Build history of the part. All positions in model axes, mm. Face numbers are marked on the shaded views. A direction names the side the tool comes from. Round coordinates to 2 decimals unless told otherwise and drop trailing zeros. Write each loop counter-clockwise with the first axis right and the second up, starting at its lowest first coordinate (ties: lowest second). Pieces come first, ordered by that corner, then holes. Notation, with made-up numbers: (20.25, 64.5) - (48.25, 64.5) arc R28 cw to (48.25, 90.5) - close; hole circle Ø2 at (24, 41.25). An arc over 180 degrees is marked (long way). One line per question, with ' | ' between items.
from build123d import *

# Parameters (mm, degrees)
F0_R     = 42
F0_R_2   = 26
F1_DEPTH = 2.5
F2_R     = 2
F3_R     = 26.5
F4_DEPTH = 45
F5_R     = 2.5
F6_T     = -0.5


# Not quite as in the source:
# - a shell that OpenCascade refuses in one call is made with other operations: the cavity is built on its own and cut out


with BuildPart() as f1:
    # F0 (on Top) → F1 (new body)
    with BuildSketch(Plane.XY):
        Circle(F0_R)
        Circle(F0_R_2, mode=Mode.SUBTRACT)
    extrude(amount=F1_DEPTH)

    # F2
    f2_edges = [f1.edges().sort_by_distance(p)[0] for p in [
        (-42, 0, 2.5),
    ]]
    fillet(f2_edges, radius=F2_R)

    # F3 (on face) → F4 (join)
    with BuildSketch(Plane(origin=(0, 0, 0), x_dir=(1, 0, 0), z_dir=(0, 0, -1))):
        Circle(F3_R)
    extrude(amount=F4_DEPTH)

    # F5
    f5_edges = [f1.edges().sort_by_distance(p)[0] for p in [
        (-26.5, 0, -45),
    ]]
    fillet(f5_edges, radius=F5_R)

    # F6: a shell. OpenCascade refuses it in one call, so the cavity is built on its own and cut out:
    # the body offset inwards by the wall thickness, plus a prism from it out through each open face.
    f6_core = offset(f1.part, amount=F6_T, kind=Kind.INTERSECTION, mode=Mode.PRIVATE)
    f6_exits = [f6_core.faces().sort_by_distance(p)[0] for p in [
        (0, 0, -0.5),
    ]]
    add(f6_core, mode=Mode.SUBTRACT)
    extrude(f6_exits, amount=-F6_T, mode=Mode.SUBTRACT)


solid = f1.part
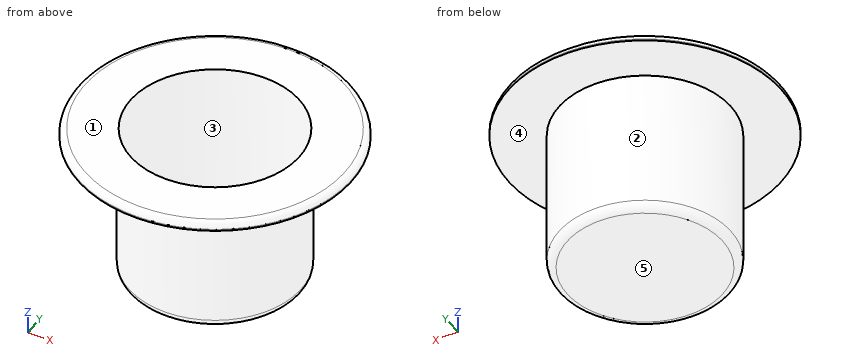
Q1. Pull direction X, two halves, no side cores. Call the marked faces 1, 2 and 3: +X half, -X half, draft (parallel to the pull), parting line (faces both ways), or undercut.
Found:
face 1: draft | face 2: parting line | face 3: undercut
Q2. Drill centre lines: L1, parallel to Y at x = 0, z = -18.5; L2, parallel to Z at x = 19, y = -19.5. Where is each one in solid material? Low to high. Write a range as from..to.
Found:
L1: -26.5..-26, 26..26.5 | L2: 0..2.5
Q3. Drop flat-ended pins along their axis: pin 1 (8 mm diameter, centred on y = 23.5, z = -9.5, fed in from -X); pin 2 (8 mm diameter, centred on y = 12.5, z = -38, fed in from +X); pin 3 (6 mm diameter, centred on y = 5.5, z = -4.5, fed in from +X). Give the stop position or say it passes through.
Found:
pin 1: x = -17.94 | pin 2: x = 25.1 | pin 3: x = 26.38
Q4. Saw through at A-A, the plane y = 0. List the corners of the cut face in (x, z), then the cut area to 3 significant figures.
Found:
outline: (-42, 0) - (-26.5, 0) - (-26.5, -42.5) arc R2.5 ccw to (-24, -45) - (24, -45) arc R2.5 ccw to (26.5, -42.5) - (26.5, 0) - (42, 0) - (42, 0.5) arc R2 ccw to (40, 2.5) - (26, 2.5) - (26, -42.5) arc R2 cw to (24, -44.5) - (-24, -44.5) arc R2 cw to (-26, -42.5) - (-26, 2.5) - (-40, 2.5) arc R2 ccw to (-42, 0.5) - close | area: 148 mm^2
Q5. Saw through at C-C, the plane z = -22. List the corners of the cut face in (x, y), then the cut area to 3 significant figures.
Found:
outline: circle Ø53 at (0, 0); hole circle Ø52 at (0, 0) | area: 82.5 mm^2
Q6. Which spindle directions (+Z, -Z, +X, -X, +Y, -Y) get a long thin tool onto all of the face, cutting with end or side? Do the marked faces 4 and 5. Say none if no direction does.
Found:
face 4: -Z | face 5: -Z, +X, -X, +Y, -Y
